from build123d import *

# Parameters (mm, degrees)
CYLINDER_R     = 3
CYLINDER_DEPTH = 3
SKETCH_R       = 1.9
PAD_DEPTH      = 5


with BuildPart() as cylinder:
    # Cylinder → Cylinder (new body)
    with BuildSketch(Plane(origin=(-6, 0, 0), x_dir=(1, 0, 0), z_dir=(0, 0, 1))):
        Circle(CYLINDER_R)
    extrude(amount=CYLINDER_DEPTH)


with BuildPart() as attach_cut:
    # Sketch → Pad (new body)
    with BuildSketch(Plane.XY):
        with BuildLine():
            Line((-6, 4.9), (6, 4.9))
            ThreePointArc((6, -4.9), (10.9, 0), (6, 4.9))
            Line((-6, -4.9), (6, -4.9))
            ThreePointArc((-6, 4.9), (-10.9, 0), (-6, -4.9))
        make_face()
        with Locations((-6, 0)):
            Circle(SKETCH_R, mode=Mode.SUBTRACT)
        with BuildLine():
            Line((-0.2, 1.9), (6, 1.9))
            ThreePointArc((6, -1.9), (7.9, 0), (6, 1.9))
            Line((-0.2, -1.9), (6, -1.9))
            ThreePointArc((-0.2, 1.9), (-2.1, 0), (-0.2, -1.9))
        make_face(mode=Mode.SUBTRACT)
    extrude(amount=PAD_DEPTH)

    # Cut: cut Cylinder
    add(cylinder.part, mode=Mode.SUBTRACT)


solid = attach_cut.part
Can you work these out from the model? Positions are in its coordinate system, mm. A direction names the side the tool comes from. Coordinates: 2 decimals unless noted, no trailing zeros. Write each loop counter-clockwise with the first axis right and the second up, starting at its lowest first coordinate (ties: lowest second). Pieces come first, ordered by that corner, then holes. Notation, with made-up numbers: M 0.25,74 L 59.25,74 A21 cw 59.25,86 Z; hole C -33.5,56 d5. An arc over 180 degrees is marked long. Use one line per item in the form item = value.
Q1. If we section it at C-C (y = 1.5): Write out the boundary of the cut face in (x, z), then the cut area to 3 significant figures.
Model answer:
outline = M -10.66,0 L -8.6,0 L -8.6,3 L -7.17,3 L -7.17,5 L -10.66,5 Z; M -4.83,3 L -3.4,3 L -3.4,0 L -1.37,0 L -1.37,5 L -4.83,5 Z; M 7.17,0 L 10.66,0 L 10.66,5 L 7.17,5 Z
area = 43.7 mm^2
Q2. I need wall thicknesses on line 1 along X through (y, z) = (0, 4.1); line 2 along Y through (x, z) = (-6, 2.2); line 3 along Y through (x, z) = (-6, 4.5). Which ranges of each line are inside material? Lowest first, please. Write a range as from..to.
Model answer:
line_1 = -10.9..-7.9, -4.1..-2.1, 7.9..10.9
line_2 = -4.9..-3, 3..4.9
line_3 = -4.9..-1.9, 1.9..4.9
Q3. We'd pull the mould along Y, two halves only. Please class faces 1 (the cylindrical face through (-7.9, 0.08, 3.99)), 2 (the cylindrical face through (10.9, -0.1, 2.5)), 3 (the flat face through (0.2, -2.1, 0)): +Y half, -Y half, draft (parallel to the pull), parting line (faces both ways), or undercut.
Model answer:
face_1 = undercut
face_2 = parting line
face_3 = draft
Q4. If we section it at D-D (x = -3.75): Write out the boundary of the cut face in (y, z), then the cut area to 3 significant figures.
Model answer:
outline = M -4.9,0 L -1.98,0 L -1.98,3 L 1.98,3 L 1.98,0 L 4.9,0 L 4.9,5 L -4.9,5 Z
area = 37.1 mm^2
Q5. For P1, Ø3, axis at x = -7, y = 1, coming from the -Z side; P2, Ø2, axis at y = 2.5, z = 1.5, coming from the +X side, each with a flat end and sliding along its axis, tell me the tip position at first contact or that it passes through.
Model answer:
P1 = 3
P2 = 10.66
Q6. For faces 4 (the cylindrical face through (-3.14, 0.9, 1.48)), 5 (the cylindrical face through (7.9, 0, 2.5)), 6 (the cylindrical face through (-10.9, 0.1, 2.5)), which set-ups out of +Z, -Z, +X, -X, +Y, -Y let a thin tool reach every point of the face, with its end or its side?
Model answer:
face_4 = -Z
face_5 = +Z, -Z
face_6 = +Z, -Z, -X
Q7. If we section it at B-B (z = 1.6): Write out the boundary of the cut face in (x, y), then the cut area to 3 significant figures.
Model answer:
outline = M -6,-4.9 L 6,-4.9 A4.9 ccw 6,4.9 L -6,4.9 A4.9 ccw Z; hole C -6,0 d6; hole M -0.2,-1.9 L 6,-1.9 A1.9 ccw 6,1.9 L -0.2,1.9 A1.9 ccw Z
area = 130 mm^2
Q8. If we section it at A-A (x = 3): Write out the boundary of the cut face in (y, z), then the cut area to 3 significant figures.
Model answer:
outline = M -4.9,0 L -1.9,0 L -1.9,5 L -4.9,5 Z; M 1.9,0 L 4.9,0 L 4.9,5 L 1.9,5 Z
area = 30.0 mm^2
